Read the model definition and answer for the solid it produces. Units are mm, in the model's axes. A direction names the side the tool comes from. Round coordinates to 2 decimals unless told otherwise and drop trailing zeros. Order: outer loops, then holes, each group sorted by start corner. A loop starts at its lowest first (then second) coordinate and runs counter-clockwise, first axis right, second up. Notation, with made-up numbers: M -14,-26.75 L -7,-26.75 A8 cw -7,-18.75 Z; hole C -8.5,-26.5 d4. An arc over 180 degrees is marked long. Answer as CSV lines item,"result".
```python
from build123d import *

# Parameters (mm, degrees)
BOSS_EXTRUDE1_DEPTH = 95
CUT_EXTRUDE1_DEPTH  = 2.2
CUT_EXTRUDE2_DEPTH  = 48.8
CUT_EXTRUDE3_DEPTH  = 2.2
SKETCH8_R           = 3.425
CUT_EXTRUDE4_DEPTH  = 50
FILLET1_R           = 1
SKETCH11_R          = 3
CUT_EXTRUDE5_DEPTH  = 15


with BuildPart() as part:
    # Sketch1 → Boss-Extrude1 (new body)
    with BuildSketch(Plane(origin=(0, 0, 0), x_dir=(1, 0, 0), z_dir=(0, 1, 0))):
        with BuildLine():
            ThreePointArc((0, 0), (14.95, 14.95), (29.9, 0))
            Line((29.9, 0), (0, 0))
        make_face()
    extrude(amount=BOSS_EXTRUDE1_DEPTH)

    # Sketch4 → Cut-Extrude1 (cut)
    with BuildSketch(Plane(origin=(0, 0, 0), x_dir=(1, 0, 0), z_dir=(0, 1, 0))):
        with BuildLine():
            Line((20.4, 0), (9.5, 0))
            ThreePointArc((9.5, 0), (14.95, 5.45), (20.4, 0))
        make_face()
    extrude(amount=CUT_EXTRUDE1_DEPTH, mode=Mode.SUBTRACT)

    # Sketch5 → Cut-Extrude2 (cut)
    with BuildSketch(Plane(origin=(0, 2.2, 0), x_dir=(-1, 0, 0), z_dir=(0, -1, 0))):
        with BuildLine():
            ThreePointArc((-12.7, 0), (-14.95, 2.25), (-17.2, 0))
            Line((-17.2, 0), (-12.7, 0))
        make_face()
        with BuildLine():
            Line((-12.7, 0), (-17.2, 0))
            ThreePointArc((-17.2, 0), (-14.95, -2.25), (-12.7, 0))
        make_face()
    extrude(amount=-CUT_EXTRUDE2_DEPTH, mode=Mode.SUBTRACT)

    # Sketch6 → Cut-Extrude3 (cut)
    with BuildSketch(Plane(origin=(0, 51, 0), x_dir=(1, 0, 0), z_dir=(0, 1, 0))):
        Polygon((25.65, 0), (4.25, 0), (4.25, 3), (14.95, 5.3), (25.65, 3), align=None)
    extrude(amount=CUT_EXTRUDE3_DEPTH, mode=Mode.SUBTRACT)

    # Sketch8 → Cut-Extrude4 (cut)
    with BuildSketch(Plane(origin=(0, 53.2, 0), x_dir=(-1, 0, 0), z_dir=(0, -1, 0))):
        with Locations((-14.95, 0)):
            Circle(SKETCH8_R)
    extrude(amount=-CUT_EXTRUDE4_DEPTH, mode=Mode.SUBTRACT)

    # Fillet1
    fillet1_edges = [part.edges().sort_by_distance(p)[0] for p in [
        (4.25, 52.1, -3),
        (25.65, 52.1, -3),
        (14.95, 52.1, -5.3),
    ]]
    fillet(fillet1_edges, radius=FILLET1_R)

    # Sketch11 → Cut-Extrude5 (cut)
    with BuildSketch(Plane.XY.offset(-0.8)):
        with Locations((5.375, 85)):
            Circle(SKETCH11_R)
        with Locations((23.125, 85)):
            Circle(SKETCH11_R)
        with Locations((5.375, 10)):
            Circle(SKETCH11_R)
        with Locations((23.125, 10)):
            Circle(SKETCH11_R)
    extrude(amount=-CUT_EXTRUDE5_DEPTH, mode=Mode.SUBTRACT)


solid = part.part
```
Item 1: Determine the mould class of faces 1 (the face through (4.25, 52, -1)), 2 (the face through (6, 47, 0)), 3 (the face through (14.621, 46.835, -14.946)), 4 (the face through (14.83, 1.08, -5.45)) for opening direction X: +X half, -X half, draft (parallel to the pull), parting line (faces both ways), or undercut.
Ans:
face 1,"undercut"
face 2,"draft"
face 3,"parting line"
face 4,"undercut"
Item 2: A cutting plane is placed at B-B, the plane y = 77. Determine the outline of the cut face in (x, z) (3 decimals), and give its area (3 significant figures).
Ans:
outline,"M 0,0 A14.95 ccw 29.9,0 L 18.375,0 A3.425 cw 11.525,0 Z"
area,"333 mm2"
Item 3: A cutting plane is placed at D-D, the plane y = 10. Determine the outline of the cut face in (x, z) (3 decimals).
Ans:
outline,"M 0,0 A14.95 ccw 2.375,-8.085 L 2.375,-0.8 L 8.375,-0.8 L 8.375,-13.427 A14.95 ccw 20.125,-14.026 L 20.125,-0.8 L 26.125,-0.8 L 26.125,-9.931 A14.95 ccw 29.9,0 L 17.2,0 A2.25 cw 12.7,0 Z"
Item 4: Find the intervals of material crossed by probe 1 along Y at (x, z) = (12.5, -3.25); probe 2 along X at (y, z) = (10, -6.5) (3 decimals); probe 3 along X at (y, z) = (85, -3.75) (3 decimals), in increasing order. Write a range as [from, to].
Ans:
probe 1,"[2.2, 51], [53.2, 95]"
probe 2,"[1.487, 2.375], [8.375, 20.125], [26.125, 28.413]"
probe 3,"[0.478, 2.375], [8.375, 20.125], [26.125, 29.422]"
Item 5: Flat-ended cylindrical pins translate along their axes: pin 1 (1.5 mm diameter, centred on y = 63, z = -4, fed in from +X); pin 2 (0.7 mm diameter, centred on y = 52, z = -1, fed in from +X); pin 3 (6.5 mm diameter, centred on x = 6.5, y = 84.5, fed in from -Z). Find the tip coordinate at first contact, or state that the pin passes through.
Ans:
pin 1,"x = 29.54"
pin 2,"x = 29.89"
pin 3,"z = -14.02"
Item 6: A tool of negligible diameter and unlimited length cuts with its end or side. For faces 5 (the face through (15, 2.2, -3)), 6 (the face through (24, 47, 0)), 7 (the face through (25.65, 52, -1)), 8 (the face through (14.875, 73.807, -3.424)), 9 (the face through (5, 10, -0.8)), from which of +Z, -Z, +X, -X, +Y, -Y can it reach the whole face along a straight path? Write none if from no direction.
Ans:
face 5,"+Z, -Y"
face 6,"+Z, +X, -X, +Y, -Y"
face 7,"+Z"
face 8,"+Z, +Y"
face 9,"-Z"
Item 7: A cutting plane is placed at A-A, the plane z = -7.75. Determine the outline of the cut face in (x, y) (3 decimals), and give its area (3 significant figures).
Ans:
outline,"M 2.166,0 L 27.734,0 L 27.734,95 L 2.166,95 Z; hole C 5.375,10 d6; hole C 5.375,85 d6; hole C 23.125,10 d6; hole C 23.125,85 d6"
area,"2,320 mm2"
Item 8: A cutting plane is placed at C-C, the plane y = 49. Determine the outline of the cut face in (x, z).
Ans:
outline,"M 0,0 A14.95 ccw 29.9,0 L 17.2,0 A2.25 cw 12.7,0 Z"
